Could you check a few things on this model? Use its own coordinates, in mm. A direction names the side the tool comes from. Coordinates: 2 decimals unless noted, no trailing zeros. Write each loop counter-clockwise with the first axis right and the second up, starting at its lowest first coordinate (ties: lowest second). Pieces come first, ordered by that corner, then holes. Notation, with made-up numbers: (2.5, -19) - (7.5, -19) arc R30 cw to (7.5, 7) - close; hole circle Ø10 at (-35.75, 61.5). An arc over 180 degrees is marked (long way). Answer as a JSON object with one key per item and string values. Group by question number.
1) Will these pins go through, and if not, where does the flat tip stop? pin 1 Ø6 at (x, y) = (-105, 1423.5) entering from +Z; pin 2 Ø10 at (x, z) = (128, 116) entering from -Y; pin 3 Ø1.5 at (y, z) = (2011.5, -33) entering from -X.
2) If we section it at A-A (z = 0): Write out the boundary of the cut face in (x, y).
3) On a 3-axis mill with a long thin cutter (end or side, diameter ignored), from which of +Z, -Z, +X, -X, +Y, -Y can I reach the whole of each face in a straight line? I mean faces 1 (the flat face through (2, 0, -2)), 2 (the flat face through (-3, 2501, -50)). Say none if no direction works.
4) If we section it at B-B (y = 244.5): Write out the boundary of the cut face in (x, z), plus the area to 3 significant figures.
5) Please list where these lines run through material, in increasing order: line 1 along Z through (x, y) = (3, 608); line 2 along X through (y, z) = (203.5, -10); line 3 along Y through (x, z) = (-108, -41).
6) We'd pull the mould along Z, two halves only. Please class faces 3 (the flat face through (-3, 2501, 50)), 4 (the flat face through (2, 2563, -97)), 5 (the conical face through (142.055, 0.971, 90.569)): released by +Z, released by -Z, zero draft, split by the parting line, or undercut.
```python
from build123d import *

# Parameters (mm, degrees)
SKETCH1_R           = 187.5
BOSS_EXTRUDE1_DEPTH = 2563
SKETCH2_W           = 375
SKETCH2_H           = 100
CUT_EXTRUDE1_DEPTH  = 125
CHAMFER1_SIZE       = 20
CHAMFER2_SIZE       = 20


with BuildPart() as part:
    # Sketch1 → Boss-Extrude1 (new body)
    with BuildSketch(Plane(origin=(0, 0, 0), x_dir=(1, 0, 0), z_dir=(0, 1, 0))):
        with Locations(Location((0, 0, 0), (0, 0, 270))):
            Circle(SKETCH1_R)
    extrude(amount=BOSS_EXTRUDE1_DEPTH)

    # Sketch2 → Cut-Extrude1 (cut)
    with BuildSketch(Plane(origin=(0, 2563, 0), x_dir=(1, 0, 0), z_dir=(0, 1, 0))):
        Rectangle(SKETCH2_W, SKETCH2_H)
    extrude(amount=-CUT_EXTRUDE1_DEPTH, mode=Mode.SUBTRACT)

    # Chamfer1
    chamfer1_edges = [part.edges().sort_by_distance(p)[0] for p in [
        (0, 2563, -187.5),
        (113.536888279, 2563, 149.216704829),
    ]]
    chamfer(chamfer1_edges, length=CHAMFER1_SIZE)

    # Chamfer2
    chamfer2_edges = [part.edges().sort_by_distance(p)[0] for p in [
        (0, 0, -187.5),
    ]]
    chamfer(chamfer2_edges, length=CHAMFER2_SIZE)


solid = part.part
```
Here are the results:
{
 "1": {"pin 1": "stops at z = 157.33", "pin 2": "stops at y = 0.24", "pin 3": "stops at x = -184.71"},
 "2": {"outline": "(-187.5, 20) - (-167.5, 0) - (167.5, 0) - (187.5, 20) - (187.5, 2438) - (-187.5, 2438) - close"},
 "3": {"face 1": "+Z, -Z, +X, -X, -Y", "face 2": "+X, -X, +Y"},
 "4": {"outline": "circle Ø375 at (0, 0)", "area": "110,000 mm²"},
 "5": {"line 1": "z = -187.48 to 187.48", "line 2": "x = -187.23 to 187.23", "line 3": "y = 0 to 2438"},
 "6": {"face 3": "undercut", "face 4": "zero draft", "face 5": "split by the parting line"}
}
